from build123d import *

# Parameters (mm, degrees)
EXTRUDE_1_DEPTH = 3
FILLET_1_R      = 0.5


with BuildPart() as part:
    # Эскиз1 → Бобышка-Вытянуть1 (new body)
    with BuildSketch(Plane.XY):
        with BuildLine():
            Line((-3, 0), (-3, 1.854101966))
            Line((-3, 1.854101966), (-2, 1.854101966))
            Line((-2, 1.854101966), (-2, 3.354101966))
            Line((-2, 3.354101966), (-3, 3.354101966))
            ThreePointArc((-3, 3.354101966), (-4.107919181, 1.837117307), (-4.5, 0))
            Line((-4.5, 0), (-4.5, -4.5))
            Line((-4.5, -4.5), (4.5, -4.5))
            Line((4.5, -4.5), (4.5, 0))
            ThreePointArc((4.5, 0), (4.107919181, 1.837117307), (3, 3.354101966))
            Line((3, 3.354101966), (2, 3.354101966))
            Line((2, 3.354101966), (2, 1.854101966))
            Line((2, 1.854101966), (3, 1.854101966))
            Line((3, 1.854101966), (3, 0))
            ThreePointArc((3, 0), (0, -3), (-3, 0))
        make_face()
    extrude(amount=EXTRUDE_1_DEPTH)

    # Скругление1
    fillet_1_edges = [part.edges().sort_by_distance(p)[0] for p in [
        (3, 1.854101966, 1.5),
        (-3, 1.854101966, 1.5),
    ]]
    fillet(fillet_1_edges, radius=FILLET_1_R)
    fillet_1_2_edges = [part.edges().sort_by_distance(p)[0] for p in [
        (3, 3.354101966, 1.5),
        (-4.5, -2.25, 0),
        (0, -4.5, 0),
        (4.5, -2.25, 0),
        (4.107919181, 1.837117307, 0),
        (2.5, 3.354101966, 0),
        (0, -3, 0),
        (-3, 0.677050983, 0),
        (-2, 2.604101966, 0),
        (-2.5, 3.354101966, 0),
        (-4.107919181, 1.837117307, 0),
        (3, 0.677050983, 0),
        (-2.5, 3.354101966, 3),
        (-2, 2.604101966, 3),
        (-3, 0.677050983, 3),
        (0, -3, 3),
        (3, 0.677050983, 3),
        (2.5, 3.354101966, 3),
        (4.107919181, 1.837117307, 3),
        (4.5, -2.25, 3),
        (0, -4.5, 3),
        (-4.5, -2.25, 3),
        (-4.107919181, 1.837117307, 3),
        (2, 3.354101966, 1.5),
        (2, 2.604101966, 3),
        (2, 1.854101966, 1.5),
        (2, 2.604101966, 0),
        (-3, 3.354101966, 1.5),
        (-2, 3.354101966, 1.5),
        (-2, 1.854101966, 1.5),
        (2.853553391, 1.707655357, 3),
        (-2.853553391, 1.707655357, 3),
        (2.853553391, 1.707655357, 0),
        (-2.853553391, 1.707655357, 0),
    ]]
    fillet(fillet_1_2_edges, radius=FILLET_1_R - 0.0001)  # a hair under: the kernel refuses the full size


solid = part.part
Source: CAD feature listing. Evaluate the final solid. Frame: model axes, mm. A direction names the side the tool comes from. Give positions to 0.01 mm unless a question says otherwise; leave off trailing zeros. Write each loop counter-clockwise with the first axis right and the second up, starting at its lowest first coordinate (ties: lowest second). Pieces come first, ordered by that corner, then holes. Notation, with made-up numbers: M 13.25,-16.5 L 39.25,-16.5 A36 ccw 39.25,18.5 Z; hole C 7,37.5 d1. An arc over 180 degrees is marked long. Return JSON: item names as keys, results as strings. Group by question number.
1) Set-up query: faces 5 (the face through (4.5, -2, 1)), 6 (the face through (-3, 1, 1)). Return all of +Z, -Z, +X, -X, +Y, -Y with unobstructed straight access to the full face (end or side cutting, diameter ignored); none if empty.
2) Pull-direction query (Y, two-part tool) for faces 1 (the face through (0, -4.5, 1)), 2 (the face through (-0.61, -3.6, 0)), 3 (the face through (0, -3, 1)), 4 (the face through (4.16, 1.72, 1.49)); classes: pulls with the +Y half, pulls with the -Y half, needs draft (parallel to the pull), parting line crosses it, or undercut.
3) Pin query (flat end, axial travel): P1, Ø1.1, axis at y = 0.5, z = 1, coming from the +X side; P2, Ø3, axis at x = 0.5, y = 2, coming from the +Z side; P3, Ø0.6, axis at y = 2.5, z = 1, coming from the -X side. Return the tip coordinate at first contact, or that it passes through.
4) Cut plane A-A, the plane x = 0. Output: boundary loops of the cut face in (y, z), plus the area to 3 significant figures.
5) Material intervals for line 1 along X through (y, z) = (2.5, 0.75); line 2 along X through (y, z) = (1.25, 1); line 3 along Y through (x, z) = (2.75, 1.35), sorted ascending. Write a range as [from, to].
Recorded:
{
 "1": {"face 5": "+Z, -Z, +X, +Y, -Y", "face 6": "+Z, -Z"},
 "2": {"face 1": "pulls with the -Y half", "face 2": "needs draft", "face 3": "undercut", "face 4": "pulls with the +Y half"},
 "3": {"P1": "stops at x = 4.5", "P2": "passes through", "P3": "stops at x = -3.93"},
 "4": {"outline": "M -4.5,0.5 A0.5 ccw -4,0 L -3.5,0 A0.5 ccw -3,0.5 L -3,2.5 A0.5 ccw -3.5,3 L -4,3 A0.5 ccw -4.5,2.5 Z", "area": "4.29 mm²"},
 "5": {"line 1": "x = [-3.74, -2], [2, 3.74]", "line 2": "x = [-4.32, -3], [3, 4.32]", "line 3": "y = [-4.5, -1.2], [1.79, 3.35]"}
}
